from build123d import *

# Parameters (mm, degrees)
PAD001_DEPTH                    = 3
PAD003_DEPTH                    = 2
PAD003_LINEARPATTERN004_2_DEPTH = 2
LINEARPATTERN005_COUNT          = 2
LINEARPATTERN005_PITCH          = 46.666667
PAD006_DEPTH                    = 4
LINEARPATTERN010_COUNT          = 2
LINEARPATTERN010_PITCH          = 56
PAD007_DEPTH                    = 4
PAD007_LINEARPATTERN011_2_DEPTH = 4


with BuildPart() as part:
    # Sketch003 → Pad001 (new body)
    with BuildSketch(Plane.XY):
        with BuildLine():
            Line((-67.8, -10.000001), (-67.8, 39.000038))
            ThreePointArc((-59.000039, 47.8), (-65.222552, 45.222551), (-67.8, 39.000038))
            Line((-59.000039, 47.8), (59.000041, 47.8))
            ThreePointArc((67.8, 39.000041), (65.22254, 45.22254), (59.000041, 47.8))
            Line((67.8, 39.000041), (67.8, -9.999998))
            ThreePointArc((30, -47.8), (56.728637, -36.728636), (67.8, -9.999998))
            Line((30, -47.8), (-29.999999, -47.8))
            ThreePointArc((-67.8, -10.000001), (-56.728636, -36.728637), (-29.999999, -47.8))
        make_face()
    extrude(amount=PAD001_DEPTH)

    # Sketch015 → Pad003 (join, symmetric)
    with BuildSketch(Plane.YZ):
        Polygon((47.8, 3), (47.8, 2), (48.8, 2), align=None)
    pad003 = extrude(amount=PAD003_DEPTH, both=True)

    # Sketch015 LinearPattern004 2 → Pad003 LinearPattern004 2 (add, symmetric)
    with BuildSketch(Plane.YZ.offset(46.666667)):
        Polygon((47.8, 3), (47.8, 2), (48.8, 2), align=None)
    pad003_linearpattern004_2 = extrude(amount=PAD003_LINEARPATTERN004_2_DEPTH, both=True)

    # LinearPattern005: Pad003, Pad003 LinearPattern004 2 ×2
    with Locations(*[(-i * LINEARPATTERN005_PITCH, 0, 0) for i in range(1, LINEARPATTERN005_COUNT)]):
        add(pad003)
        add(pad003_linearpattern004_2)

    # Sketch020 → Pad006 (join)
    with BuildSketch(Plane.YZ.offset(-30)):
        Polygon((-47.8, 3), (-47.8, 2), (-48.8, 2), align=None)
    pad006 = extrude(amount=PAD006_DEPTH)

    # LinearPattern010: Pad006 ×2
    with Locations(*[(i * LINEARPATTERN010_PITCH, 0, 0) for i in range(1, LINEARPATTERN010_COUNT)]):
        add(pad006)

    # Sketch021 → Pad007 (join)
    with BuildSketch(Plane.XZ.offset(10)):
        Polygon((68.8, 2), (67.8, 2), (67.8, 3), align=None)
    pad007 = extrude(amount=-PAD007_DEPTH)

    # Sketch021 LinearPattern011 2 → Pad007 LinearPattern011 2 (add)
    with BuildSketch(Plane.XZ.offset(-28)):
        Polygon((68.8, 2), (67.8, 2), (67.8, 3), align=None)
    pad007_linearpattern011_2 = extrude(amount=-PAD007_LINEARPATTERN011_2_DEPTH)

    # Mirrored004: Pad007, Pad007 LinearPattern011 2 across Sketch021 V_Axis
    add(pad007.mirror(Plane(origin=(0, -10, 0), x_dir=(0, -1, 0), z_dir=(1, 0, 0))))
    add(pad007_linearpattern011_2.mirror(Plane(origin=(0, -10, 0), x_dir=(0, -1, 0), z_dir=(1, 0, 0))))


solid = part.part
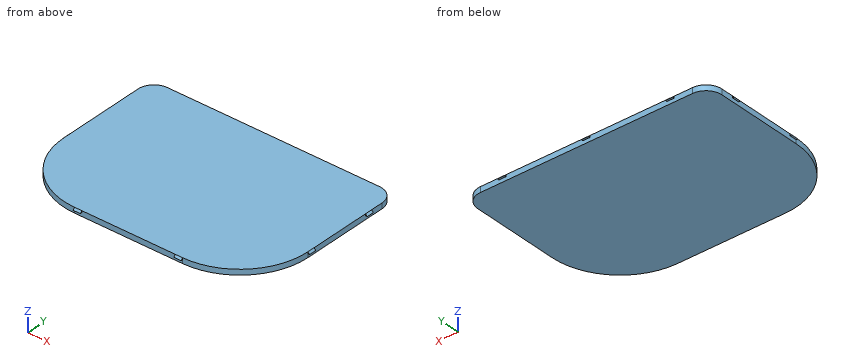
Here's how the part is built. I have some questions about the finished solid (model axes, mm). Round coordinates to 2 decimals unless told otherwise and drop trailing zeros. Loops run counter-clockwise (first coordinate to the right, second up) from the corner with the lowest first, then second, coordinate; pieces in that order, holes last. Notation, with made-up numbers: M 69.5,-25 L 128.5,-25 A21 cw 128.5,3 Z; hole C 79,54 d9. An arc over 180 degrees is marked long. Write each question's results on one line, items separated by ' | '. Start each with the question number.
(1) I want a section at D-D (x = 21.5). Please give me the cut outline in (y, z), then the cut area to 3 significant figures.
(2) If I drill on probe 1 along X at (y, z) = (24, 2.3); probe 2 along Y at (x, z) = (-20, 1.7); probe 3 along Y at (x, z) = (-36, 2.8), over which ranges is the centre line in solid material (lowest first)? Write a range as from..to.
(3) I want a section at C-C (y = -34). Please give me the cut outline in (x, z), then the cut area to 3 significant figures.
(4) I want a section at B-B (x = -28). Please give me the cut outline in (y, z).
(5) Will these pins go through, and if not, where does the flat tip stop? P1, Ø0.8, axis at x = -46.5, y = 48.5, coming from the -Z side; P2, Ø0.5, axis at x = -68.5, z = 2.5, coming from the -Y side; P3, Ø1.5, axis at x = -40, z = 0.5, coming from the -Y side.
(6) I want a section at A-A (z = 1.1). Please give me the cut outline in (x, y).
Solved:
1) outline: M -47.8,0 L 47.8,0 L 47.8,3 L -47.8,3 Z | area: 287 mm²
2) probe 1: x = -67.8..67.8 | probe 2: y = -47.8..47.8 | probe 3: y = -47.32..47.8
3) outline: M -59.2,0 L 59.2,0 L 59.2,3 L -59.2,3 Z | area: 355 mm²
4) outline: M -48.8,2 L -47.8,2 L -47.8,0 L 47.8,0 L 47.8,3 L -47.8,3 Z
5) P1: stops at z = 2 | P2: stops at y = -10 | P3: stops at y = -46.65
6) outline: M -67.8,-10 A37.8 ccw -30,-47.8 L 30,-47.8 A37.8 ccw 67.8,-10 L 67.8,39 A8.8 ccw 59,47.8 L -59,47.8 A8.8 ccw -67.8,39 Z
